Answer from the drawing. Dimensions are ordinates in mm from the lowest x, y and z of the part. A direction names the side the tool comes from. Coordinates: 2 decimals unless noted, no trailing zeros. Order: outer loops, then holes, each group sorted by start corner. A loop starts at its lowest first (then second) coordinate and runs counter-clockwise, first axis right, second up. Notation, with made-up numbers: (25, -5.5) - (36, -5.5) arc R21 cw to (36, 28.5) - close; hole circle Ø6 at (31, 51). An arc over 180 degrees is marked (long way). Answer as a JSON object with one key per item and string values. Group by question number.
1) Find the intervals of material crossed by line 1 along Y through (x, z) = (15.5, 5.25); line 2 along X through (y, z) = (16.5, 4); line 3 along Z through (x, y) = (27, 8.5), in increasing order.
2) The mould has two halves that part along Y. Classify the marked faces 3, 4 and 5: released by +Y, released by -Y, zero draft, split by the parting line, or undercut.
3) Section A-A (x = 22.5) is taken. Give the vertices of the cut face in (y, z), plus the area to 3 significant figures.
4) Each of these flat-tipped pins is pushed along its axis until it touches: P1, Ø5, axis at y = 17, z = 7.5, coming from the -X side; P2, Ø1, axis at x = 24.5, y = 14.5, coming from the +Z side. Where does it stop, or does it pass through?
5) Section B-B (y = 2.25) is taken. Give the vertices of the cut face in (x, z), plus the area to 3 significant figures.
6) A tool of negligible diameter and unlimited length cuts with its end or side. For the marked faces 1 and 2, from which of +Z, -Z, +X, -X, +Y, -Y can it reach the whole face along a straight path? Write none if from no direction.
7) Section C-C (z = 7.25) is taken. Give the vertices of the cut face in (x, y).
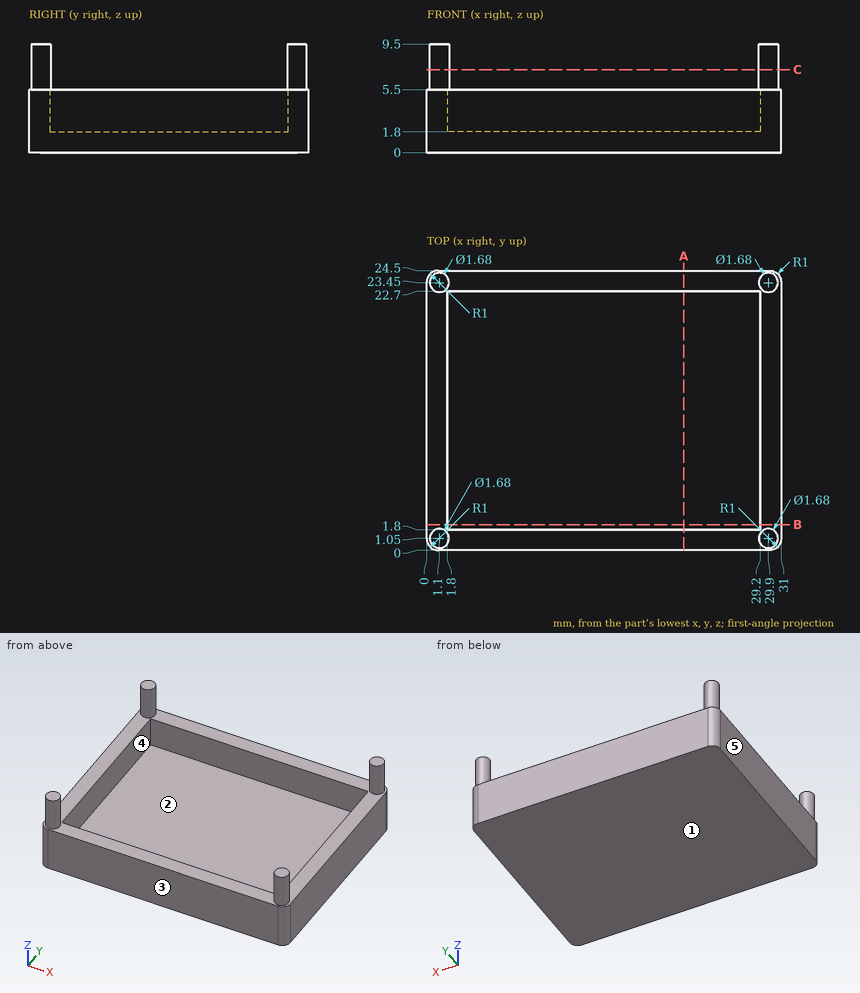
Report:
{
 "1": {"line 1": "y = 0 to 1.8, 22.7 to 24.5", "line 2": "x = 0 to 1.8, 29.2 to 31", "line 3": "z = 0 to 1.8"},
 "2": {"face 3": "released by -Y", "face 4": "undercut", "face 5": "zero draft"},
 "3": {"outline": "(0, 0) - (24.5, 0) - (24.5, 5.5) - (22.7, 5.5) - (22.7, 1.8) - (1.8, 1.8) - (1.8, 5.5) - (0, 5.5) - close", "area": "57.4 mm²"},
 "4": {"P1": "stops at x = 0", "P2": "stops at z = 1.8"},
 "5": {"outline": "(0, 0) - (31, 0) - (31, 5.5) - (29.2, 5.5) - (29.2, 1.8) - (1.8, 1.8) - (1.8, 5.5) - (0, 5.5) - close", "area": "69.1 mm²"},
 "6": {"face 1": "-Z, +X, -X, +Y, -Y", "face 2": "+Z"},
 "7": {"outline": "circle Ø1.68 at (1.1, 1.05); circle Ø1.68 at (1.1, 23.45); circle Ø1.68 at (29.9, 1.05); circle Ø1.68 at (29.9, 23.45)"}
}
